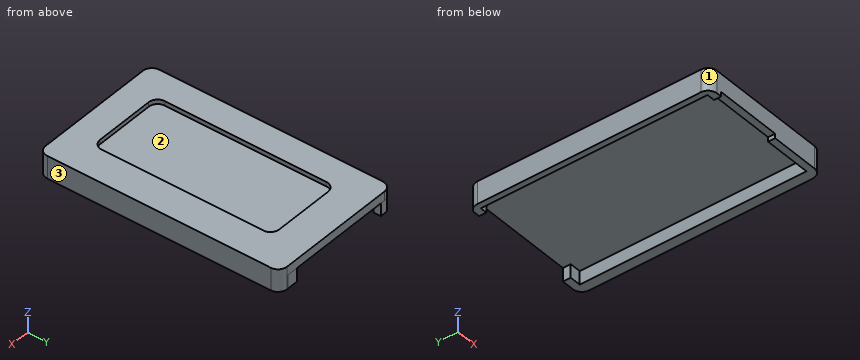
```python
from build123d import *

# Parameters (mm, degrees)
SKETCH_5_W          = 31
SKETCH_5_H          = 53.868777402
SKETCH_5_W_2        = 27.381586342
SKETCH_5_H_2        = 50.42341648
EXTRUDE_3_DEPTH     = 3
SKETCH_8_W          = 15
SKETCH_8_H          = 1.581115617
CUT_EXTRUDE_6_DEPTH = 1
SKETCH_9_W          = 31
SKETCH_9_H          = 53.868777402
EXTRUDE_5_DEPTH     = 2
SKETCH_10_W         = 17.475002228
SKETCH_10_H         = 39.986467982
CUT_EXTRUDE_7_DEPTH = 1
FILLET_1_R          = 2
FILLET_2_R          = 2
SKETCH_11_W         = 27.381586342
SKETCH_11_H         = 3
CUT_EXTRUDE_8_DEPTH = 2
SKETCH_14_W         = 2.490628955
SKETCH_14_H         = 1.721797648
SKETCH_14_W_2       = 1.5
SKETCH_14_H_2       = 1.606542801
EXTRUDE_6_DEPTH     = 3


with BuildPart() as part:
    # 草图5 → 凸台-拉伸3 (new body)
    with BuildSketch(Plane.XY.offset(15)):
        with Locations((52.576231829, -51.822040042)):
            Rectangle(SKETCH_5_W, SKETCH_5_H)
        with Locations((52.104679946, -51.963604886)):
            Rectangle(SKETCH_5_W_2, SKETCH_5_H_2, mode=Mode.SUBTRACT)
    extrude(amount=EXTRUDE_3_DEPTH)

    # 草图8 → 切除-拉伸6 (cut)
    with BuildSketch(Plane(origin=(0, 0, 15), x_dir=(-1, 0, 0), z_dir=(0, 0, -1))):
        with Locations((-47.690080224, -77.965870935)):
            Rectangle(SKETCH_8_W, SKETCH_8_H)
    extrude(amount=-CUT_EXTRUDE_6_DEPTH, mode=Mode.SUBTRACT)

    # 草图9 → 凸台-拉伸5 (add)
    with BuildSketch(Plane.XY.offset(18)):
        with Locations((52.576231829, -51.822040042)):
            Rectangle(SKETCH_9_W, SKETCH_9_H)
    extrude(amount=EXTRUDE_5_DEPTH)

    # 草图10 → 切除-拉伸7 (cut)
    with BuildSketch(Plane.XY.offset(20)):
        with Locations((52.039568352, -52.470675496)):
            Rectangle(SKETCH_10_W, SKETCH_10_H)
    extrude(amount=-CUT_EXTRUDE_7_DEPTH, mode=Mode.SUBTRACT)

    # 圆角1
    fillet_1_edges = [part.edges().sort_by_distance(p)[0] for p in [
        (37.076231829, -78.756428743, 17.5),
        (37.076231829, -24.887651341, 17.5),
        (68.076231829, -24.887651341, 17.5),
        (68.076231829, -78.756428743, 17.5),
    ]]
    fillet(fillet_1_edges, radius=FILLET_1_R)

    # 圆角2
    fillet_2_edges = [part.edges().sort_by_distance(p)[0] for p in [
        (43.302067238, -72.463909487, 19.5),
        (43.302067238, -32.477441505, 19.5),
        (60.777069466, -32.477441505, 19.5),
        (60.777069466, -72.463909487, 19.5),
    ]]
    fillet(fillet_2_edges, radius=FILLET_2_R)

    # 草图11 → 切除-拉伸8 (cut)
    with BuildSketch(Plane(origin=(0, -26.751896646, 0), x_dir=(-1, 0, 0), z_dir=(0, -1, 0))):
        with Locations((-52.104679946, -16.5)):
            Rectangle(SKETCH_11_W, SKETCH_11_H)
    extrude(amount=-CUT_EXTRUDE_8_DEPTH, mode=Mode.SUBTRACT)

    # 草图14 → 凸台-拉伸6 (add)
    with BuildSketch(Plane(origin=(0, 0, 18), x_dir=(-1, 0, 0), z_dir=(0, 0, -1))):
        with Locations((-64.550158639, -25.755243126)):
            Rectangle(SKETCH_14_W, SKETCH_14_H)
        with Locations((-39.163886775, -25.81287055)):
            Rectangle(SKETCH_14_W_2, SKETCH_14_H_2)
    extrude(amount=EXTRUDE_6_DEPTH)


solid = part.part
```
CAD build for the part. Positions are in the model's coordinates, mm. Face numbers are marked on the shaded views. Give positions to 0.01 mm unless a question says otherwise; leave off trailing zeros. Write each loop counter-clockwise with the first axis right and the second up, starting at its lowest first coordinate (ties: lowest second). Pieces come first, ordered by that corner, then holes. Notation, with made-up numbers: (-26, 18.5) -> (9, 18.5) arc R38 ccw to (9, 56.5) -> close; hole circle Ø8 at (28.5, -26). An arc over 180 degrees is marked (long way). Write each question's results on one line, items separated by ' | '.
1. Drop flat-ended pins along their axis: P1, Ø0.5, axis at x = 47, y = -77.5, coming from the -Z side; P2, Ø6, axis at x = 45, y = -41, coming from the -Z side; P3, Ø0.7, axis at x = 64.5, z = 16.5, coming from the +Y side. Give the stop position or say it passes through.
Geometry check:
P1: z = 16 | P2: z = 18 | P3: y = -24.89
2. Cut at D-D, the plane x = 54. Write the cut outline in (y, z).
Geometry check:
outline: (-78.76, 16) -> (-77.18, 16) -> (-77.18, 18) -> (-24.89, 18) -> (-24.89, 20) -> (-32.48, 20) -> (-32.48, 19) -> (-72.46, 19) -> (-72.46, 20) -> (-78.76, 20) -> close
3. Two-plate mould, pull along Y, no slides. Class the marked faces 1, 2 and 3: pulls with the +Y half, pulls with the -Y half, needs draft (parallel to the pull), parting line crosses it, or undercut.
Geometry check:
face 1: pulls with the -Y half | face 2: undercut | face 3: needs draft
4. Cut at C-C, the plane y = -36. Write the cut outline in (x, z), then the cut area to 3 significant figures.
Geometry check:
outline: (37.08, 15) -> (38.41, 15) -> (38.41, 18) -> (65.8, 18) -> (65.8, 15) -> (68.08, 15) -> (68.08, 20) -> (60.78, 20) -> (60.78, 19) -> (43.3, 19) -> (43.3, 20) -> (37.08, 20) -> close | area: 55.4 mm²
5. Wall check: probe 1 along X at (y, z) = (-46, 17.9); probe 2 along Y at (x, z) = (64.5, 17.3); probe 3 along X at (y, z) = (-56, 19.7). Give the ranges that are in metal, low to high. Write a range as [from, to].
Geometry check:
probe 1: [37.08, 38.41], [65.8, 68.08] | probe 2: [-78.76, -77.18], [-26.62, -24.89] | probe 3: [37.08, 43.3], [60.78, 68.08]
6. Cut at B-B, the plane x = 62. Write the cut outline in (y, z), then the cut area to 3 significant figures.
Geometry check:
outline: (-78.76, 15) -> (-77.18, 15) -> (-77.18, 18) -> (-24.89, 18) -> (-24.89, 20) -> (-78.76, 20) -> close | area: 112 mm²
